Check sheet for the modelled part. Datum: model origin and axes. Units: mm. A direction names the side the tool comes from. Round coordinates to 2 decimals unless told otherwise and drop trailing zeros. Write each loop counter-clockwise with the first axis right and the second up, starting at its lowest first coordinate (ties: lowest second). Pieces come first, ordered by that corner, then holes. Notation, with made-up numbers: M 34.5,-12 L 43.5,-12 A11 cw 43.5,-6 Z; hole C 31,-15.5 d2. An arc over 180 degrees is marked long. Put each result on its own line as item: value.
Autodesk Inventor part; units mm, degrees
ref_plane "РабПлоскость1" through (-243.8305, -139, 0) normal (0, 1, 0) x (-1, 0, 0)
ref_plane "YZ Plane" through (0, 0, 0) normal (1, 0, 0) x (0, 1, 0)
ref_plane "XZ Plane" through (0, 0, 0) normal (0, 1, 0) x (-1, 0, 0)
ref_plane "РабПлоскость1" through (-243.8305, -139, 0) normal (0, 1, 0) x (-1, 0, 0)
sketch "Эскиз1" plane through (-243.8305, -139, 0) normal (0, 1, 0) x (-1, 0, 0)
  line L0 (-217.7305, 128) -> (-241.9805, 128)
  line L1 (-241.9805, 128) -> (-241.9805, 134)
  line L2 (-217.7305, 134) -> (-241.9805, 134)
  line L3 (-217.7305, 128) -> (-217.7305, 134) construction
  line L4 (-218.8555, 120) -> (-240.8555, 120)
  line L5 (-243.8555, 123) -> (-243.8555, 139)
  line L6 (-240.8555, 142) -> (-218.8555, 142)
  line L7 (-215.8555, 139) -> (-215.8555, 123)
  line L8 (-229.8555, 128) -> (-229.8555, 134) construction
  line L9 (-217.7305, 131) -> (-241.9805, 131) construction
  line L10 (-238.8555, 138) -> (-220.8555, 138) construction
  line L11 (-220.8555, 138) -> (-220.8555, 124) construction
  line L12 (-220.8555, 124) -> (-238.8555, 124) construction
  line L13 (-238.8555, 124) -> (-238.8555, 138) construction
  line L14 (-238.8555, 138) -> (-220.8555, 124) construction
  line L15 (-220.8555, 138) -> (-238.8555, 124) construction
  circle A0 centre (-220.8555, 124) radius 1.95
  circle A1 centre (-238.8555, 124) radius 1.95
  circle A2 centre (-238.8555, 138) radius 1.95
  circle A3 centre (-220.8555, 138) radius 1.95
  arc A4 (-218.8555, 120) -> (-215.8555, 123) centre (-218.8555, 123) ccw
  arc A5 (-215.8555, 139) -> (-218.8555, 142) centre (-218.8555, 139) ccw
  arc A6 (-240.8555, 142) -> (-243.8555, 139) centre (-240.8555, 139) ccw
  arc A7 (-243.8555, 123) -> (-240.8555, 120) centre (-240.8555, 123) ccw
  line L16 (-217.7305, 128) -> (-215.8555, 128)
  line L17 (-215.8555, 128) -> (-215.8555, 134)
  line L18 (-215.8555, 134) -> (-217.7305, 134)
  line L19 (-217.7305, 134) -> (-217.7305, 128) construction
  point P0 (-243.8305, 0)
  point P1 (-243.8555, 142)
  point P2 (-243.8555, 120)
  point P3 (-215.8555, 142)
  point P4 (-229.8555, 131)
  dimension "d0" = 28
  dimension "d1" = 22
  dimension "d2" = 3.9
  dimension "d3" = 18
  dimension "d4" = 14
  dimension "d5" = 3
extrude "Выдавливание1" add sketch "Эскиз1" along normal blind 10 contours L16 L7 A4 L4 A7 L5 A6 L6 A5 L18 L2 L1 L0
chamfer "Фаска1" distance 2 angle 45 2 edges at (-27.975, -134, 134) (-27.975, -134, 128)
properties part number "Фиксатор_сервопривода" material "По умолчанию1"
1. Cross-section at D-D (z = 130.5). Enter the section's corners in (x, y) (3 decimals).
Computed values:
outline: M -1.85,-139 L 0.025,-139 L 0.025,-129 L -1.85,-129 Z
2. Depth check by flat-ended pin: pin 1 Ø3 at (x, z) = (-18, 130.5) entering from +Y; pin 2 Ø1.5 at (y, z) = (-133, 133.5) entering from -X (3 decimals); pin 3 Ø3 at (y, z) = (-135.5, 130.5) entering from -X. Enter the tip coordinate at first touch or a pass-through.
Computed values:
pin 1: passes through
pin 2: stops at x = -26.225
pin 3: stops at x = -1.85
3. Cross-section at A-A (x = -18.25). Enter the section's corners in (y, z).
Computed values:
outline: M -139,120 L -129,120 L -129,128 L -139,128 Z; M -139,134 L -129,134 L -129,142 L -139,142 Z
4. Access from +Z, -Z, +X, -X, +Y, -Y to the whole of each face (thin tool, end or side, straight path). Record for faces 1 (the flat face through (-1.85, -134, 131)), 2 (the flat face through (0.025, -134, 131)).
Computed values:
face 1: -X, +Y, -Y
face 2: +Z, -Z, +X, +Y, -Y
5. Release check for a two-part mould opening along X. For faces 3 (the cylindrical face through (-4.721, -134.07, 136.067)), 4 (the flat face through (-14, -139, 126)), 5 (the cylindrical face through (-0.83, -134.07, 141.1)) record: +X half, -X half, draft (parallel to the pull), parting line (faces both ways), or undercut.
Computed values:
face 3: undercut
face 4: draft
face 5: +X half
6. Cross-section at C-C (x = -23.5). Enter the section's corners in (y, z).
Computed values:
outline: M -139,120 L -129,120 L -129,122.12 L -139,122.12 Z; M -139,125.88 L -129,125.88 L -129,128 L -139,128 Z; M -139,134 L -129,134 L -129,136.12 L -139,136.12 Z; M -139,139.88 L -129,139.88 L -129,142 L -139,142 Z
7. Scan lines: probe 1 along X at (y, z) = (-131, 138) (3 decimals); probe 2 along Z at (x, y) = (-20, -131.75); probe 3 along Z at (x, y) = (-23, -134.5). Record each from-to range of solid material in increasing order.
Computed values:
probe 1: x = -27.975 to -24.925, -21.025 to -6.925, -3.025 to 0.025
probe 2: z = 120 to 128, 134 to 142
probe 3: z = 120 to 122.05, 125.95 to 128, 134 to 136.05, 139.95 to 142
8. Cross-section at B-B (z = 138). Enter the section's corners in (x, y) (3 decimals).
Computed values:
outline: M -27.975,-139 L -24.925,-139 L -24.925,-129 L -27.975,-129 Z; M -21.025,-139 L -6.925,-139 L -6.925,-129 L -21.025,-129 Z; M -3.025,-139 L 0.025,-139 L 0.025,-129 L -3.025,-129 Z
